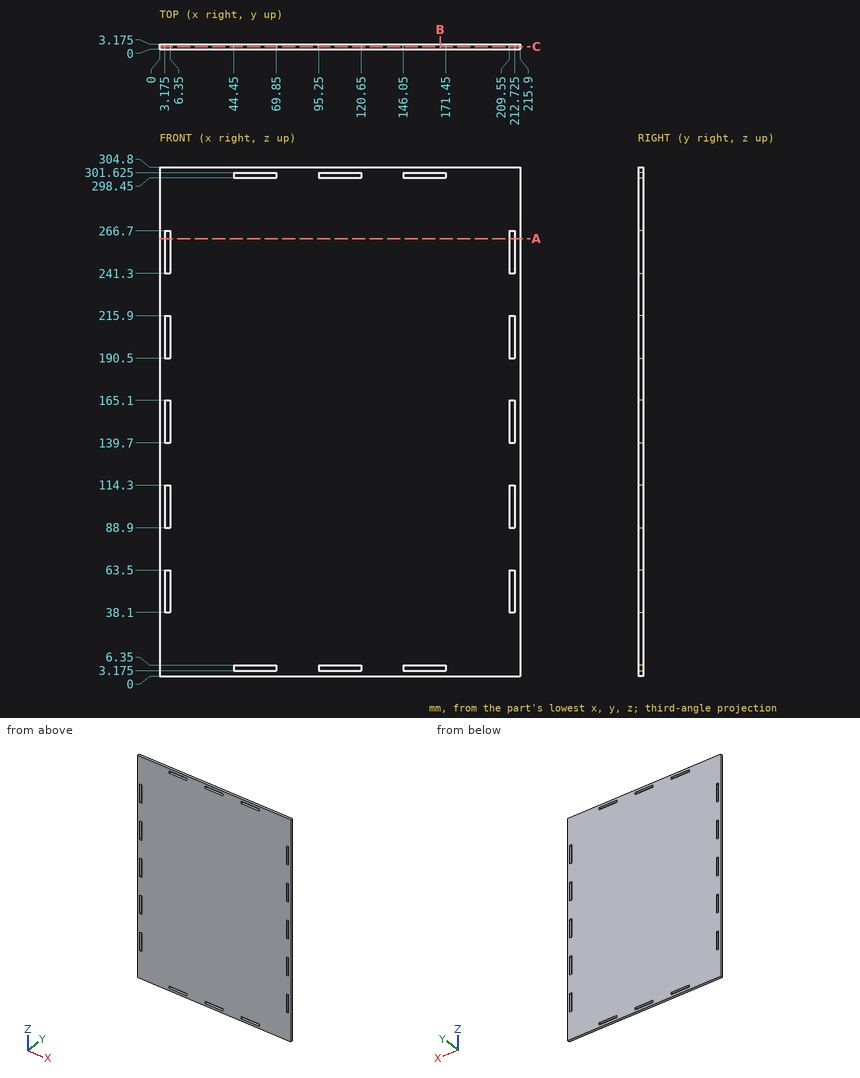
Answer from the drawing. Dimensions are ordinates in mm from the lowest x, y and z of the part. Give positions to 0.01 mm unless a question says otherwise; leave off trailing zeros. Write each loop counter-clockwise with the first axis right and the second up, starting at its lowest first coordinate (ties: lowest second). Pieces come first, ordered by that corner, then holes. Notation, with made-up numbers: (47, 9) - (90, 9) arc R31 cw to (90, 41) - close; hole circle Ø2 at (54.5, 71.5). An arc over 180 degrees is marked (long way). Answer in a Markdown table with one row per item. Add a question column.
Item 1: Section A-A, the plane z = 262 is taken. Write down the section's boundary in (x, y) (3 decimals), and give its area (3 significant figures).
Item 2: Section B-B, the plane x = 168 is taken. Write down the section's boundary in (y, z) (3 decimals), and give its area (3 significant figures).
Item 3: Find the intervals of material crossed by L1, parallel to Z at x = 157, y = 0.35 (3 decimals); L2, parallel to X at y = 1.9, z = 250 (3 decimals), in increasing order.
Item 4: A flat-ended cylindrical pin translates along its axis: P1, Ø1.6, axis at x = 212, y = 2, coming from the -Z side. Find the tip coordinate at first contact, or state that the pin passes through.
Item 5: Section C-C, the plane y = 1.65 is taken. Count the separate pieces of the cut face and the enclosed holes in it, and give its area (3 significant figures).
Recorded:
| question | item | result |
|---|---|---|
| 1 | outline | (0, 0) - (3.175, 0) - (3.175, 3.175) - (0, 3.175) - close; (6.35, 0) - (209.55, 0) - (209.55, 3.175) - (6.35, 3.175) - close; (212.725, 0) - (215.9, 0) - (215.9, 3.175) - (212.725, 3.175) - close |
| 1 | area | 665 mm2 |
| 2 | outline | (0, 0) - (3.175, 0) - (3.175, 3.175) - (0, 3.175) - close; (0, 6.35) - (3.175, 6.35) - (3.175, 298.45) - (0, 298.45) - close; (0, 301.625) - (3.175, 301.625) - (3.175, 304.8) - (0, 304.8) - close |
| 2 | area | 948 mm2 |
| 3 | L1 | z = 0 to 3.175, 6.35 to 298.45, 301.625 to 304.8 |
| 3 | L2 | x = 0 to 3.175, 6.35 to 209.55, 212.725 to 215.9 |
| 4 | P1 | stops at z = 0 |
| 5 | separate pieces | 1 |
| 5 | enclosed holes | 16 |
| 5 | area | 64,500 mm2 |
